```python
from build123d import *

# Parameters (mm, degrees)
SKIZZE1_W                       = 11
SKIZZE1_H                       = 60
SKIZZE1_H_2                     = 15
SKIZZE1_W_2                     = 48
AUFSATZ_LINEAR_AUSTRAGEN1_DEPTH = 5
SKIZZE2_R                       = 1.65
SCHNITT_LINEAR_AUSTRAGEN1_DEPTH = 5
SKIZZE6_W                       = 70
SKIZZE6_H                       = 5
AUFSATZ_LINEAR_AUSTRAGEN3_DEPTH = 10
SKIZZE7_R                       = 1.65
SCHNITT_LINEAR_AUSTRAGEN2_DEPTH = 10


with BuildPart() as part:
    # Skizze1 → Aufsatz-Linear austragen1 (new body)
    with BuildSketch(Plane.XY):
        with Locations((-29.5, 37.5)):
            Rectangle(SKIZZE1_W, SKIZZE1_H)
        with Locations((-29.5, 0)):
            Rectangle(SKIZZE1_W, SKIZZE1_H_2)
        Rectangle(SKIZZE1_W_2, SKIZZE1_H_2)
        with Locations((29.5, 0)):
            Rectangle(SKIZZE1_W, SKIZZE1_H_2)
        with Locations((29.5, 37.5)):
            Rectangle(SKIZZE1_W, SKIZZE1_H)
    extrude(amount=AUFSATZ_LINEAR_AUSTRAGEN1_DEPTH)

    # Skizze2 → Schnitt-Linear austragen1 (cut)
    with BuildSketch(Plane.XY.offset(5)):
        with Locations((-27.997843094, 3.700522334)):
            Circle(SKIZZE2_R)
        with Locations((27.502156906, 3.700522334)):
            Circle(SKIZZE2_R)
        with Locations((27.75, 62.5)):
            Circle(SKIZZE2_R)
        with Locations((-27.75, 62.5)):
            Circle(SKIZZE2_R)
    extrude(amount=-SCHNITT_LINEAR_AUSTRAGEN1_DEPTH, mode=Mode.SUBTRACT)

    # Skizze6 → Aufsatz-Linear austragen3 (add)
    with BuildSketch(Plane.XY.offset(5)):
        with Locations((0, -5)):
            Rectangle(SKIZZE6_W, SKIZZE6_H)
    extrude(amount=AUFSATZ_LINEAR_AUSTRAGEN3_DEPTH)

    # Skizze7 → Schnitt-Linear austragen2 (cut)
    with BuildSketch(Plane(origin=(0, -2.5, 0), x_dir=(1, 0, 0), z_dir=(0, 1, 0))):
        with Locations((-27.75, -10)):
            Circle(SKIZZE7_R)
        with Locations((27.75, -10)):
            Circle(SKIZZE7_R)
    extrude(amount=-SCHNITT_LINEAR_AUSTRAGEN2_DEPTH, mode=Mode.SUBTRACT)


solid = part.part
```
Check sheet for the modelled part. Datum: model origin and axes. Units: mm. A direction names the side the tool comes from. Give positions to 0.01 mm unless a question says otherwise; leave off trailing zeros. Write each loop counter-clockwise with the first axis right and the second up, starting at its lowest first coordinate (ties: lowest second). Pieces come first, ordered by that corner, then holes. Notation, with made-up numbers: (4, 41) -> (8, 41) arc R23 cw to (8, 57) -> close; hole circle Ø4 at (-23, 43). An arc over 180 degrees is marked (long way). Use CSV: the item, a comma, the result in double quotes. Start each with the question number.
Q1. Scan lines: line 1 along X through (y, z) = (-6.25, 10); line 2 along Y through (x, z) = (-27.75, 1.1); line 3 along Z through (x, y) = (-27.75, -4.85). Record each from-to range of solid material in increasing order.
Q2. Cross-section at C-C on y = 20.5. Enter the section's corners in (x, z), and give its area (3 significant figures).
Q3. Cross-section at D-D on x = 27.75. Enter the section's corners in (y, z).
Q4. Depth check by flat-ended pin: P1, Ø2, axis at x = 27.5, y = 3.7, coming from the -Z side; P2, Ø2, axis at x = 17.5, z = 11.5, coming from the +Y side; P3, Ø8, axis at x = 12, z = 8, coming from the +Y side; P4, Ø6, axis at x = -22, y = 21, coming from the +Z side. Enter the tip coordinate at first touch or a pass-through.
Q5. Cross-section at B-B on y = 62.5. Enter the section's corners in (x, z).
Q6. Cross-section at A-A on z = 10. Enter the section's corners in (x, y), and give its area (3 significant figures).
Q7. Tool access check on faces 1 (the flat face through (0, -2.5, 10)), 2 (the flat face through (24, 37, 2)), 3 (the cylindrical face through (-29.06, -4.96, 11)). Record the directions out of +Z, -Z, +X, -X, +Y, -Y that give a thin tool (end or side, any length) a straight path to the whole face; none if there is none.
Q8. Release check for a two-part mould opening along X. For faces 4 (the flat face through (29, 67.5, 2)), 5 (the cylindrical face through (29.076, 4.196, 2.535)), 6 (the flat face through (35, 21, 4)), 7 (the flat face through (-35, 21, 4)) record: +X half, -X half, draft (parallel to the pull), parting line (faces both ways), or undercut.
Working result:
1,line 1,"x = -35 to -29.4, -26.1 to 26.1, 29.4 to 35"
1,line 2,"y = -7.5 to 2.07, 5.33 to 60.85, 64.15 to 67.5"
1,line 3,"z = 0 to 8.35, 11.65 to 15"
2,outline,"(-35, 0) -> (-24, 0) -> (-24, 5) -> (-35, 5) -> close; (24, 0) -> (35, 0) -> (35, 5) -> (24, 5) -> close"
2,area,"110 mm^2"
3,outline,"(-7.5, 0) -> (2.07, 0) -> (2.07, 5) -> (-2.5, 5) -> (-2.5, 8.35) -> (-7.5, 8.35) -> close; (-7.5, 11.65) -> (-2.5, 11.65) -> (-2.5, 15) -> (-7.5, 15) -> close; (5.33, 0) -> (60.85, 0) -> (60.85, 5) -> (5.33, 5) -> close; (64.15, 0) -> (67.5, 0) -> (67.5, 5) -> (64.15, 5) -> close"
4,P1,"passes through"
4,P2,"stops at y = -2.5"
4,P3,"stops at y = 7.5"
4,P4,"stops at z = 5"
5,outline,"(-35, 0) -> (-29.4, 0) -> (-29.4, 5) -> (-35, 5) -> close; (-26.1, 0) -> (-24, 0) -> (-24, 5) -> (-26.1, 5) -> close; (24, 0) -> (26.1, 0) -> (26.1, 5) -> (24, 5) -> close; (29.4, 0) -> (35, 0) -> (35, 5) -> (29.4, 5) -> close"
6,outline,"(-35, -7.5) -> (-29.4, -7.5) -> (-29.4, -2.5) -> (-35, -2.5) -> close; (-26.1, -7.5) -> (26.1, -7.5) -> (26.1, -2.5) -> (-26.1, -2.5) -> close; (29.4, -7.5) -> (35, -7.5) -> (35, -2.5) -> (29.4, -2.5) -> close"
6,area,"317 mm^2"
7,face 1,"+Z, +X, -X, +Y"
7,face 2,"+Z, -Z, +Y"
7,face 3,"+Y, -Y"
8,face 4,"draft"
8,face 5,"undercut"
8,face 6,"+X half"
8,face 7,"-X half"
